The model under review builds one solid part; all positions refer to its coordinate system, in mm. Round coordinates to 2 decimals unless told otherwise and drop trailing zeros. Loops run counter-clockwise (first coordinate to the right, second up) from the corner with the lowest first, then second, coordinate; pieces in that order, holes last. Notation, with made-up numbers: M 3,46 L 56,46 A23 ccw 56,73 Z; hole C 71.25,82.5 d7. An arc over 180 degrees is marked long. One line per question, with ' | ' between items.
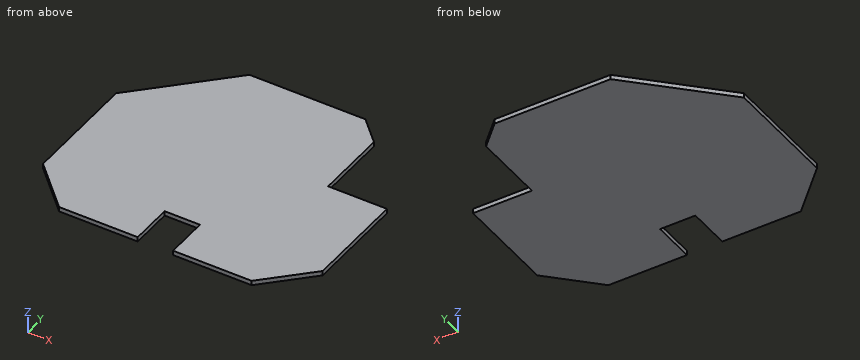
Autodesk Inventor part; units mm, degrees
ref_plane "YZ Plane" through (0, 0, 0) normal (1, 0, 0) x (0, 1, 0)
ref_plane "XZ Plane" through (0, 0, 0) normal (0, 1, 0) x (-1, 0, 0)
ref_plane "XY Plane" through (0, 0, 0) normal (0, 0, 1) x (1, 0, 0)
sketch "Sketch1" plane through (0, 0, 0) normal (0, 0, 1) x (1, 0, 0)
  line L0 (0, 0) -> (0, 24.8008)
  line L1 (0, 0) -> (23.5103, 0)
  line L2 (-19.7, 47.5) -> (19.7, 47.5)
  line L3 (47.5, 19.7) -> (47.5, -19.7)
  line L4 (19.7, -47.5) -> (-19.7, -47.5)
  line L5 (-47.5, -19.7) -> (-47.5, 19.7)
  line L6 (19.7, 47.5) -> (47.5, 19.7)
  line L7 (47.5, -19.7) -> (19.7, -47.5)
  line L8 (-19.7, -47.5) -> (-47.5, -19.7)
  line L9 (-47.5, 19.7) -> (-19.7, 47.5)
  point P0 (-47.5, 47.5)
  point P1 (47.5, -47.5)
  point P2 (47.5, 47.5)
  point P3 (-47.5, -47.5)
  dimension "d9" = 27.8
  dimension "d10" = 27.8
  dimension "d11" = 27.8
  dimension "d12" = 27.8
  dimension "d13" = 27.8
  dimension "d14" = 27.8
  dimension "d15" = 27.8
  dimension "d16" = 27.8
  dimension "d17" = 95
  dimension "d18" = 95
extrude "Extrusion1" add sketch "Sketch1" along normal mid plane 1.5748
sketch "Sketch4" plane through (0, 0, 0.7874) normal (0, 0, 1) x (1, 0, 0)
  line L0 (19.7, -47.5) -> (-19.7, -47.5)
  line L1 (-35, -47.5) -> (35, -47.5)
  line L2 (35, -47.5) -> (35, -34.5)
  line L3 (35, -34.5) -> (-35, -34.5)
  line L4 (-35, -34.5) -> (-35, -47.5)
  point P0 (12, -47.5)
  point P1 (0, 0)
  point P2 (0, -34.5)
  dimension "d24" = 13
  dimension "d25" = 70
extrude "Extrusion4" cut sketch "Sketch4" against normal through all
sketch "Sketch5" plane through (0, 0, 0.7874) normal (0, 0, 1) x (1, 0, 0)
  line L0 (-6, -47.5) -> (6, -47.5)
  line L1 (6, -47.5) -> (6, -20)
  line L2 (6, -20) -> (-6, -20)
  line L3 (-6, -20) -> (-6, -47.5)
  line L4 (0, 0) -> (0, -10.8647)
  dimension "d29" = 12
  dimension "d30" = 27.5
  dimension "d45" = 20
extrude "Extrusion5" cut sketch "Sketch5" against normal through all
sketch "Sketch7" plane through (0, 0, -0.7874) normal (0, 0, -1) x (-1, 0, 0)
  line L0 (-47.5, -19.7) -> (-47.5, 19.7)
  line L1 (-47.5, 40) -> (-27.5, 40)
  line L2 (-27.5, 40) -> (-27.5, 15)
  line L3 (-27.5, 15) -> (-47.5, 15)
  line L4 (-47.5, 15) -> (-47.5, 40)
  point P0 (0, 0)
  point P1 (-27.5, 27.5)
  point P2 (-27.5, 27.5)
  dimension "d37" = 25
  dimension "d38" = 20
  dimension "d46" = 15
extrude "Extrusion7" cut sketch "Sketch7" against normal through all
properties part number "Pb_TX_bot" material "Lead"
1) Insertion check: P1, Ø0.8, axis at x = 36.5, z = 0, coming from the +Y side. The pin has a flat end and moves straight along its axis. Give the tip position at first contact, or say it passes through.
Output values:
P1: stops at y = 15
2) Add section D-D on y = 16.5. State the section outline as (x, z) points.
Output values:
outline: M -47.5,-0.79 L 27.5,-0.79 L 27.5,0.79 L -47.5,0.79 Z
3) Add section C-C on x = -22. State the section outline as (y, z) points.
Output values:
outline: M -34.5,-0.79 L 45.2,-0.79 L 45.2,0.79 L -34.5,0.79 Z
4) For line 1 (Y direction, x = -2, z = 0.45); line 2 (X direction, y = 19.5, z = -0.4); line 3 (X direction, y = -26, z = 0.05), list the stretches that pass through material, from the lowest coordinate up.
Output values:
line 1: y = -20 to 47.5 | line 2: x = -47.5 to 27.5 | line 3: x = -41.2 to -6, 6 to 41.2
5) Add section B-B on z = 0.3. State the section outline as (x, y) points, then the cut area to 3 significant figures.
Output values:
outline: M -47.5,-19.7 L -32.7,-34.5 L -6,-34.5 L -6,-20 L 6,-20 L 6,-34.5 L 32.7,-34.5 L 47.5,-19.7 L 47.5,15 L 27.5,15 L 27.5,39.7 L 19.7,47.5 L -19.7,47.5 L -47.5,19.7 Z | area: 6,330 mm²
6) Add section A-A on y = -29.5. State the section outline as (x, z) points, then the cut area to 3 significant figures.
Output values:
outline: M -37.7,-0.79 L -6,-0.79 L -6,0.79 L -37.7,0.79 Z; M 6,-0.79 L 37.7,-0.79 L 37.7,0.79 L 6,0.79 Z | area: 99.8 mm²
